from build123d import *

# Parameters (mm, degrees)
SKETCH1_W           = 180
SKETCH1_H           = 57.2
SKETCH1_W_2         = 50
SKETCH1_H_2         = 15
BOSS_EXTRUDE1_DEPTH = 36.2
SKETCH2_R           = 3.25
SKETCH2_R_2         = 5.75
SKETCH2_R_3         = 1.75
CUT_EXTRUDE1_DEPTH  = 57.2
FILLET1_R           = 7.5
CUT_EXTRUDE3_START  = -52.2
SKETCH3_R           = 1.75
SKETCH3_R_2         = 5.75
CUT_EXTRUDE3_DEPTH  = 52.2
SKETCH4_W           = 42.5
SKETCH4_H           = 42.5
SKETCH4_R           = 11.25
SKETCH4_R_2         = 1.75
CUT_EXTRUDE4_DEPTH  = 33.2
SKETCH4_3_R         = 11.25
SKETCH4_3_R_2       = 1.75
CUT_EXTRUDE5_DEPTH  = 36.2
FILLET2_R           = 7.5
SKETCH8_R           = 3
CUT_EXTRUDE8_DEPTH  = 1.5
SKETCH7_R           = 3.25
CUT_EXTRUDE7_DEPTH  = 36.2
SKETCH7_2_R         = 3.25
BOSS_EXTRUDE3_DEPTH = 22.4
CUT_EXTRUDE9_REACH  = 190.71
SKETCH9_W           = 16.2
SKETCH9_H           = 28


with BuildPart() as part:
    # Sketch1 → Boss-Extrude1 (new body)
    with BuildSketch(Plane.XY):
        Rectangle(SKETCH1_W, SKETCH1_H)
        with Locations((50, 36.1)):
            Rectangle(SKETCH1_W_2, SKETCH1_H_2)
    extrude(amount=BOSS_EXTRUDE1_DEPTH)

    # Sketch2 → Cut-Extrude1 (cut)
    with BuildSketch(Plane.XZ.offset(28.6)):
        with Locations(Location((-82.5, 14, 0), (0, 0, 270))):
            Circle(SKETCH2_R)
        with Locations(Location((-32.25, 14, 0), (0, 0, 270))):
            Circle(SKETCH2_R_2)
        with Locations(Location((-37.906854249, 19.656854249, 0), (0, 0, 270))):
            Circle(SKETCH2_R_3)
        with Locations(Location((-26.593145751, 19.656854249, 0), (0, 0, 270))):
            Circle(SKETCH2_R_3)
        with Locations(Location((-37.906854249, 8.343145751, 0), (0, 0, 270))):
            Circle(SKETCH2_R_3)
        with Locations(Location((-26.593145751, 8.343145751, 0), (0, 0, 270))):
            Circle(SKETCH2_R_3)
        with Locations(Location((82.5, 14, 0), (0, 0, 270))):
            Circle(SKETCH2_R)
    extrude(amount=-CUT_EXTRUDE1_DEPTH, mode=Mode.SUBTRACT)

    # Fillet1
    fillet1_edges = [part.edges().sort_by_distance(p)[0] for p in [
        (-90, 0, 0),
        (90, 0, 0),
        (-90, 0, 36.2),
        (90, 0, 36.2),
    ]]
    fillet(fillet1_edges, radius=FILLET1_R)

    # Sketch3 → Cut-Extrude3 (cut)
    with BuildSketch(Plane(origin=(0, 28.6, 0), x_dir=(1, 0, 0), z_dir=(0, 1, 0)).offset(CUT_EXTRUDE3_START)):
        with BuildLine():
            Line((-40.382558646, -6.593145751), (-70, -6.593145751))
            ThreePointArc((-70, -6.593145751), (-73.535533906, -8.057611845), (-75, -11.593145751))
            Line((-75, -11.593145751), (-75, -27.6))
            ThreePointArc((-75, -27.6), (-73.535533906, -31.135533906), (-70, -32.6))
            Line((-70, -32.6), (25, -32.6))
            Line((25, -32.6), (25, -6.593145751))
            Line((25, -6.593145751), (-24.117441354, -6.593145751))
            ThreePointArc((-24.117441354, -6.593145751), (-32.25, -3), (-40.382558646, -6.593145751))
        make_face()
        with Locations(Location((-26.593145751, -8.343145751, 0), (0, 0, 90))):
            Circle(SKETCH3_R, mode=Mode.SUBTRACT)
        with Locations(Location((-37.906854249, -19.656854249, 0), (0, 0, 90))):
            Circle(SKETCH3_R, mode=Mode.SUBTRACT)
        with Locations(Location((-26.593145751, -19.656854249, 0), (0, 0, 90))):
            Circle(SKETCH3_R, mode=Mode.SUBTRACT)
        with Locations(Location((-37.906854249, -8.343145751, 0), (0, 0, 90))):
            Circle(SKETCH3_R, mode=Mode.SUBTRACT)
        with Locations(Location((-32.25, -14, 0), (0, 0, 90))):
            Circle(SKETCH3_R_2, mode=Mode.SUBTRACT)
    extrude(amount=CUT_EXTRUDE3_DEPTH, mode=Mode.SUBTRACT)

    # Sketch4 → Cut-Extrude4 (cut)
    with BuildSketch(Plane.XY.offset(36.2)):
        with Locations((50, 7.35)):
            Rectangle(SKETCH4_W, SKETCH4_H)
        with Locations((50, 7.35)):
            Circle(SKETCH4_R, mode=Mode.SUBTRACT)
        with Locations((34.5, 22.85)):
            Circle(SKETCH4_R_2, mode=Mode.SUBTRACT)
        with Locations((65.5, 22.85)):
            Circle(SKETCH4_R_2, mode=Mode.SUBTRACT)
        with Locations((65.5, -8.15)):
            Circle(SKETCH4_R_2, mode=Mode.SUBTRACT)
        with Locations((34.5, -8.15)):
            Circle(SKETCH4_R_2, mode=Mode.SUBTRACT)
    extrude(amount=-CUT_EXTRUDE4_DEPTH, mode=Mode.SUBTRACT)

    # Sketch4<3> → Cut-Extrude5 (cut)
    with BuildSketch(Plane.XY.offset(36.2)):
        with Locations((50, 7.35)):
            Circle(SKETCH4_3_R)
        with Locations((34.5, 22.85)):
            Circle(SKETCH4_3_R_2)
        with Locations((65.5, 22.85)):
            Circle(SKETCH4_3_R_2)
        with Locations((65.5, -8.15)):
            Circle(SKETCH4_3_R_2)
        with Locations((34.5, -8.15)):
            Circle(SKETCH4_3_R_2)
    extrude(amount=-CUT_EXTRUDE5_DEPTH, mode=Mode.SUBTRACT)

    # Fillet2
    fillet2_edges = [part.edges().sort_by_distance(p)[0] for p in [
        (25, 43.6, 18.1),
        (75, 43.6, 18.1),
    ]]
    fillet(fillet2_edges, radius=FILLET2_R)

    # Sketch8 → Cut-Extrude8 (cut)
    with BuildSketch(Plane(origin=(0, 0, 0), x_dir=(-1, 0, 0), z_dir=(0, 0, -1))):
        with Locations((-65.5, 22.85)):
            Circle(SKETCH8_R)
        with Locations((-34.5, 22.85)):
            Circle(SKETCH8_R)
        with Locations((-34.5, -8.15)):
            Circle(SKETCH8_R)
        with Locations((-65.5, -8.15)):
            Circle(SKETCH8_R)
    extrude(amount=-CUT_EXTRUDE8_DEPTH, mode=Mode.SUBTRACT)

    # Sketch7 → Cut-Extrude7 (cut)
    with BuildSketch(Plane.XY.offset(36.2)):
        with Locations((50, -21.4)):
            Circle(SKETCH7_R)
        with Locations((50, 36.1)):
            Circle(SKETCH7_R)
    extrude(amount=-CUT_EXTRUDE7_DEPTH, mode=Mode.SUBTRACT)

    # Sketch7<2> → Boss-Extrude3 (add)
    with BuildSketch(Plane.XY.offset(36.2)):
        with Locations((50, -21.4)):
            Circle(SKETCH7_2_R)
        with Locations((50, 36.1)):
            Circle(SKETCH7_2_R)
    extrude(amount=-BOSS_EXTRUDE3_DEPTH)

    # Cut-Extrude9: up to this face of the body (flat: up to its plane)
    cut_extrude9_end = Plane(part.part.faces().sort_by_distance((71.25, 7.35, 19.6))[0])
    # Sketch9 → Cut-Extrude9 (cut, up to the picked face)
    with BuildSketch(Plane(origin=(90, 0, 0), x_dir=(0, 0, -1), z_dir=(1, 0, 0)), mode=Mode.PRIVATE) as cut_extrude9_sk1:
        with Locations((-28.1, 7.35)):
            Rectangle(SKETCH9_W, SKETCH9_H)
    cut_extrude9_tool1 = split(extrude(cut_extrude9_sk1.sketch, amount=-CUT_EXTRUDE9_REACH, mode=Mode.PRIVATE), bisect_by=cut_extrude9_end, keep=Keep.BOTH, mode=Mode.PRIVATE)
    add(cut_extrude9_tool1.solids().sort_by(Axis((90, 7.35, 28.1), (-1, 0, 0)))[0], mode=Mode.SUBTRACT)


solid = part.part
The model under review builds one solid part; all positions refer to its coordinate system, in mm. A direction names the side the tool comes from. Coordinates: 2 decimals unless noted, no trailing zeros. Loops run counter-clockwise (first coordinate to the right, second up) from the corner with the lowest first, then second, coordinate; pieces in that order, holes last.
(1) Consider section D-D, the plane y = -21.4. Give the boundary of the cut face in (x, z), plus the area to 3 significant figures.
Determined:
outline: (-90, 7.5) arc R7.5 ccw to (-82.5, 0) - (46.75, 0) - (46.75, 13.8) - (53.25, 13.8) - (53.25, 0) - (82.5, 0) arc R7.5 ccw to (90, 7.5) - (90, 28.7) arc R7.5 ccw to (82.5, 36.2) - (-82.5, 36.2) arc R7.5 ccw to (-90, 28.7) - close; hole circle Ø6.5 at (-82.5, 14); hole (-75, 11.59) arc R5 ccw to (-70, 6.59) - (-40.38, 6.59) arc R11 ccw to (-24.12, 6.59) - (25, 6.59) - (25, 32.6) - (-70, 32.6) arc R5 ccw to (-75, 27.6) - close; hole circle Ø6.5 at (82.5, 14)
area: 3,680 mm2
(2) Draft analysis for pull direction Y (two halves, no side actions). For faces 4 (the cylindrical face through (-24.858, -26.135, 8.571)), 5 (the flat face through (63.5, -8.1, 1.5)), 6 (the cylindrical face through (72.861, 41.345, 18.353)), state which applies: +Y half, -Y half, draft (parallel to the pull), parting line (faces both ways), or undercut.
Determined:
face 4: draft
face 5: undercut
face 6: +Y half
(3) Consider section C-C, the plane x = 65.5. Give the boundary of the cut face in (y, z), plus the area to 3 significant figures.
Determined:
outline: (-28.6, 0) - (-11.15, 0) - (-11.15, 1.5) - (-9.9, 1.5) - (-9.9, 3) - (-13.9, 3) - (-13.9, 36.2) - (-28.6, 36.2) - close; (-6.4, 1.5) - (-5.15, 1.5) - (-5.15, 0) - (19.85, 0) - (19.85, 1.5) - (21.1, 1.5) - (21.1, 3) - (-6.4, 3) - close; (24.6, 1.5) - (25.85, 1.5) - (25.85, 0) - (43.6, 0) - (43.6, 36.2) - (28.6, 36.2) - (28.6, 3) - (24.6, 3) - close
area: 1,170 mm2
(4) Wall thickness on L1, parallel to Y at x = 65.5, z = 1.95; L2, parallel to X at y = -14, z = 24; L3, parallel to Z at x = 13, y = -18: over which ranges is each line inside the solid? List them lowest first.
Determined:
L1: y = -28.6 to -9.9, -6.4 to 21.1, 24.6 to 43.6
L2: x = -90 to -75, 25 to 90
L3: z = 0 to 6.59, 32.6 to 36.2
(5) Tool access review of faces 1 (the flat face through (71.25, 7, 16)), 2 (the flat face through (81, 21.35, 28)), 3 (the flat face through (50, 36, 13.8)): name each direction out of +Z, -Z, +X, -X, +Y, -Y from which nothing blocks a thin tool from reaching the whole face with its end or side.
Determined:
face 1: +Z
face 2: +Z, +X
face 3: -Z
(6) Insertion check: P1, Ø4.5, axis at x = -37.91, z = 8.34, coming from the +Y side; P2, Ø12, axis at x = 57.5, y = 14.5, coming from the +Z side; P3, Ø5.5, axis at x = 65.5, y = 22.85, coming from the -Z side. Each pin has a flat end and moves straight along its axis. Give the tip position at first contact, or say it passes through.
Determined:
P1: stops at y = -23.6
P2: stops at z = 3
P3: stops at z = 1.5
(7) Consider section B-B, the plane y = 10. Give the boundary of the cut face in (x, z).
Determined:
outline: (-90, 7.5) arc R7.5 ccw to (-82.5, 0) - (39.07, 0) - (39.07, 3) - (28.75, 3) - (28.75, 36.2) - (-82.5, 36.2) arc R7.5 ccw to (-90, 28.7) - close; (60.93, 0) - (82.5, 0) arc R7.5 ccw to (90, 7.5) - (90, 20) - (71.25, 20) - (71.25, 3) - (60.93, 3) - close; hole circle Ø6.5 at (-82.5, 14); hole (-75, 11.59) arc R5 ccw to (-70, 6.59) - (-40.38, 6.59) arc R11 ccw to (-24.12, 6.59) - (25, 6.59) - (25, 32.6) - (-70, 32.6) arc R5 ccw to (-75, 27.6) - close; hole circle Ø6.5 at (82.5, 14)
(8) Consider section A-A, the plane x = -32.25. Give the boundary of the cut face in (y, z).
Determined:
outline: (-28.6, 0) - (28.6, 0) - (28.6, 3) - (-23.6, 3) - (-23.6, 8.25) - (-28.6, 8.25) - close; (-28.6, 19.75) - (-23.6, 19.75) - (-23.6, 32.6) - (28.6, 32.6) - (28.6, 36.2) - (-28.6, 36.2) - close
